Geometry: final body of the model. Coordinates: model frame, mm. A direction names the side the tool comes from. Coordinates: 2 decimals unless noted, no trailing zeros. Loops run counter-clockwise (first coordinate to the right, second up) from the corner with the lowest first, then second, coordinate; pieces in that order, holes last. Notation, with made-up numbers: (-2, -12) - (35, -12) arc R12 ccw to (35, -5) - close; hole circle Ø1 at (36.5, 86.5). An arc over 180 degrees is marked (long way). Answer in a Markdown table with one row per item.
from build123d import *

# Parameters (mm, degrees)
F0_W     = 69.85
F0_H     = 100
F1_DEPTH = 12.5
F2_R     = 1.25
F2_W     = 53.85
F2_H     = 5
F3_DEPTH = 6
F4_R     = 1.25
F5_DEPTH = 3


# Not quite as in the source:
# - a pattern or mirror of a feature is missing from the dataset's text; its kind, count and spacing are read off the source's solid


with BuildPart() as f1:
    # F0 (on Front) → F1 (new body)
    with BuildSketch(Plane.XZ):
        with Locations((34.925, 50)):
            Rectangle(F0_W, F0_H)
    extrude(amount=F1_DEPTH)

    # F2 (on face) → F3 (cut)
    with BuildSketch(Plane.XZ.offset(12.5)):
        with Locations((4.065, 9.4)):
            Circle(F2_R)
        with Locations((4.065, 86)):
            Circle(F2_R)
        with Locations((65.785, 9.4)):
            Circle(F2_R)
        with Locations((65.785, 86)):
            Circle(F2_R)
        with Locations((34.925, 97.5)):
            Rectangle(F2_W, F2_H)
    extrude(amount=-F3_DEPTH, mode=Mode.SUBTRACT)

    # F4 (on face) → F5 (cut)
    with BuildSketch(Plane(origin=(0, 0, 0), x_dir=(0, -1, 0), z_dir=(-1, 0, 0))):
        with Locations((9.5, 86)):
            Circle(F4_R)
        with Locations((9.5, 9.4)):
            Circle(F4_R)
    f5 = extrude(amount=-F5_DEPTH, mode=Mode.SUBTRACT)

    # F5_copies: F5 across plane
    add(f5.mirror(Plane(origin=(34.925, 0, 0), x_dir=(0, 0, 1), z_dir=(1, 0, 0))), mode=Mode.SUBTRACT)


solid = f1.part
(1) Ray query, probe 1 along X at (y, z) = (-8.1, 86) (3 decimals); probe 2 along Z at (x, y) = (1.1, -9.5); probe 3 along Y at (x, z) = (2, 86). Return the intervals inside material, ascending.
Verdict:
| item | result |
|---|---|
| probe 1 | x = 0 to 2.815, 5.315 to 64.535, 67.035 to 69.85 |
| probe 2 | z = 0 to 8.15, 10.65 to 84.75, 87.25 to 100 |
| probe 3 | y = -12.5 to -10.75, -8.25 to 0 |
(2) Access query for faces 1 (the face through (66, -6.5, 9)), 2 (the face through (1.48, -8.25, 9.45)), 3 (the face through (68.37, -9.34, 87.24)), 4 (the face through (61.85, -10, 97)). Directions: +Z, -Z, +X, -X, +Y, -Y. A direction counts if a zero-diameter tool reaches every point of the face in a straight line with its end or side. Return the directions, or none.
Verdict:
| item | result |
|---|---|
| face 1 | -Y |
| face 2 | -X |
| face 3 | +X |
| face 4 | +Z, -Y |
(3) Pull-direction query (X, two-part tool) for faces 5 (the face through (0, -6, 49)), 6 (the face through (35, -6.5, 98)), 7 (the face through (68.37, -8.25, 9.45)); classes: pulls with the +X half, pulls with the -X half, needs draft (parallel to the pull), parting line crosses it, or undercut.
Verdict:
| item | result |
|---|---|
| face 5 | pulls with the -X half |
| face 6 | undercut |
| face 7 | needs draft |
(4) First-contact query: pin 1 Ø6 at (x, y) = (33, -7) entering from -Z; pin 2 Ø2 at (x, z) = (4.065, 9.4) entering from -Y; pin 3 Ø1.5 at (y, z) = (-9.5, 86) entering from +X. Flat tips, straight axial feed; report the tip coordinate or a pass-through.
Verdict:
| item | result |
|---|---|
| pin 1 | stops at z = 0 |
| pin 2 | stops at y = -6.5 |
| pin 3 | stops at x = 66.85 |
(5) Cut plane B-B on x = 30. Output: boundary loops of the cut face in (y, z).
Verdict:
| item | result |
|---|---|
| outline | (-12.5, 0) - (0, 0) - (0, 100) - (-6.5, 100) - (-6.5, 95) - (-12.5, 95) - close |
